from build123d import *

# Parameters (mm, degrees)
F0_W     = 9
F0_H     = 139.6909442604
F0_R     = 1.5
F0_H_2   = 81.4090557396
F1_DEPTH = 10


with BuildPart() as f1:
    # F0 (on Top) → F1 (new body)
    with BuildSketch(Plane.XY):
        with Locations((-251.2277567387, 73.9804314047)):
            Rectangle(F0_W, F0_H)
        with Locations((-251.2277567387, 18.8259035349)):
            Circle(F0_R, mode=Mode.SUBTRACT)
        with Locations((-251.2277567387, 38.8259035349)):
            Circle(F0_R, mode=Mode.SUBTRACT)
        with Locations((-251.2277567387, 58.8259035349)):
            Circle(F0_R, mode=Mode.SUBTRACT)
        with Locations((-251.2277567387, 78.8259035349)):
            Circle(F0_R, mode=Mode.SUBTRACT)
        with Locations((-251.2277567387, 98.8259035349)):
            Circle(F0_R, mode=Mode.SUBTRACT)
        with Locations((-251.2277567387, 118.8259035349)):
            Circle(F0_R, mode=Mode.SUBTRACT)
        with Locations((-251.2277567387, 138.8259035349)):
            Circle(F0_R, mode=Mode.SUBTRACT)
        with BuildLine():
            Line((-246.7277567387, 4.1349592745), (-255.7277567387, 4.1349592745))
            Line((-255.7277567387, 4.1349592745), (-255.7277567387, -3.9008271631))
            ThreePointArc((-255.7277567387, -3.9008271631), (-255.0030118673, -4.4490153217), (-254.7277567387, -5.3150407255))
            ThreePointArc((-254.7277567387, -5.3150407255), (-255.0030118673, -6.1810661293), (-255.7277567387, -6.7292542878))
            Line((-255.7277567387, -6.7292542878), (-255.7277567387, -13.9008271631))
            ThreePointArc((-255.7277567387, -13.9008271631), (-255.0030118673, -14.4490153217), (-254.7277567387, -15.3150407255))
            ThreePointArc((-254.7277567387, -15.3150407255), (-255.0030118673, -16.1810661293), (-255.7277567387, -16.7292542878))
            Line((-255.7277567387, -16.7292542878), (-255.7277567387, -24.7650407255))
            Line((-255.7277567387, -24.7650407255), (-246.7277567387, -24.7650407255))
            Line((-246.7277567387, -24.7650407255), (-246.7277567387, -16.7292542878))
            ThreePointArc((-246.7277567387, -16.7292542878), (-247.7277567387, -15.3150407255), (-246.7277567387, -13.9008271631))
            Line((-246.7277567387, -13.9008271631), (-246.7277567387, -6.7292542878))
            ThreePointArc((-246.7277567387, -6.7292542878), (-247.7277567387, -5.3150407255), (-246.7277567387, -3.9008271631))
            Line((-246.7277567387, -3.9008271631), (-246.7277567387, 4.1349592745))
        make_face()
        with Locations((-251.2277567387, -21.1740964651)):
            Circle(F0_R, mode=Mode.SUBTRACT)
        with Locations((-251.2277567387, -1.1740964651)):
            Circle(F0_R, mode=Mode.SUBTRACT)
        with BuildLine():
            Line((-255.7277567387, -3.9008271631), (-255.7277567387, 4.1349592745))
            Line((-255.7277567387, 4.1349592745), (-261.2277567387, 4.1349592745))
            Line((-261.2277567387, 4.1349592745), (-261.2277567387, -24.7650407255))
            Line((-261.2277567387, -24.7650407255), (-255.7277567387, -24.7650407255))
            Line((-255.7277567387, -24.7650407255), (-255.7277567387, -16.7292542878))
            ThreePointArc((-255.7277567387, -16.7292542878), (-257.7277567387, -15.3150407255), (-255.7277567387, -13.9008271631))
            Line((-255.7277567387, -13.9008271631), (-255.7277567387, -6.7292542878))
            ThreePointArc((-255.7277567387, -6.7292542878), (-257.7277567387, -5.3150407255), (-255.7277567387, -3.9008271631))
        make_face()
        with BuildLine():
            Line((-241.2277567387, 4.1349592745), (-246.7277567387, 4.1349592745))
            Line((-246.7277567387, 4.1349592745), (-246.7277567387, -3.9008271631))
            ThreePointArc((-246.7277567387, -3.9008271631), (-245.3617313349, -4.0902958541), (-244.7277567387, -5.3150407255))
            ThreePointArc((-244.7277567387, -5.3150407255), (-245.3617313349, -6.5397855969), (-246.7277567387, -6.7292542878))
            Line((-246.7277567387, -6.7292542878), (-246.7277567387, -13.9008271631))
            ThreePointArc((-246.7277567387, -13.9008271631), (-245.3617313349, -14.0902958541), (-244.7277567387, -15.3150407255))
            ThreePointArc((-244.7277567387, -15.3150407255), (-245.3617313349, -16.5397855969), (-246.7277567387, -16.7292542878))
            Line((-246.7277567387, -16.7292542878), (-246.7277567387, -24.7650407255))
            Line((-246.7277567387, -24.7650407255), (-241.2277567387, -24.7650407255))
            Line((-241.2277567387, -24.7650407255), (-241.2277567387, 4.1349592745))
        make_face()
        with Locations((-251.2277567387, -65.4695685953)):
            Rectangle(F0_W, F0_H_2)
        with Locations((-251.3328434825, -101.1740964651)):
            Circle(F0_R, mode=Mode.SUBTRACT)
        with Locations((-251.2277567387, -81.1740964651)):
            Circle(F0_R, mode=Mode.SUBTRACT)
        with Locations((-251.2277567387, -61.1740964651)):
            Circle(F0_R, mode=Mode.SUBTRACT)
        with Locations((-251.2277567387, -41.1740964651)):
            Circle(F0_R, mode=Mode.SUBTRACT)
    extrude(amount=F1_DEPTH)


solid = f1.part
Verification items for the finished model (mm, model axes). A direction names the side the tool comes from. Give positions to 0.01 mm unless a question says otherwise; leave off trailing zeros. Order: outer loops, then holes, each group sorted by start corner. A loop starts at its lowest first (then second) coordinate and runs counter-clockwise, first axis right, second up. Notation, with made-up numbers: M -30,-34.5 L -7,-34.5 A32 cw -7,3.5 Z; hole C 41,-23 d1. An arc over 180 degrees is marked long. Answer as a JSON object with one key per item and string values. Group by question number.
1) Cross-section at B-B (z = 3.25). Give the number of separate pieces and of enclosed holes in the cut face, then the cut area to 3 significant figures.
2) Cross-section at A-A (y = -53). Enter the section's corners in (x, z).
3) Access from +Z, -Z, +X, -X, +Y, -Y to the whole of each face (thin tool, end or side, straight path). Record for faces 1 (the face through (-255.728, -66, 5)), 2 (the face through (-258, 4.135, 5)), 3 (the face through (-244, 4.135, 5)), 4 (the face through (-251, 21, 0)), 5 (the face through (-246.728, -66, 5)).
4) Scan lines: line 1 along X through (y, z) = (79, 3.5); line 2 along Y through (x, z) = (-257, 2.25); line 3 along Y through (x, z) = (-245.25, 9.5). Record each from-to range of solid material in increasing order. Write a range as [from, to].
5) Depth check by flat-ended pin: pin 1 Ø2.5 at (x, y) = (-251.23, 138.83) entering from +Z; pin 2 Ø2 at (y, z) = (94, 7.5) entering from -X; pin 3 Ø1.5 at (x, z) = (-259, 1.5) entering from -Y; pin 4 Ø4 at (y, z) = (-62, 2.5) entering from +X. Enter the tip coordinate at first touch or a pass-through.
Result sheet:
{
 "1": {"separate pieces": "1", "enclosed holes": "17", "area": "2,450 mm2"},
 "2": {"outline": "M -255.73,0 L -246.73,0 L -246.73,10 L -255.73,10 Z"},
 "3": {"face 1": "+Z, -Z, -X, -Y", "face 2": "+Z, -Z, -X, +Y", "face 3": "+Z, -Z, +X, +Y", "face 4": "-Z, +X, -X, +Y, -Y", "face 5": "+Z, -Z, +X, -Y"},
 "4": {"line 1": "x = [-255.73, -252.72], [-249.74, -246.73]", "line 2": "y = [-24.77, -16.6], [-14.03, -6.6], [-4.03, 4.13]", "line 3": "y = [-24.77, -16.45], [-14.18, -6.45], [-4.18, 4.13]"},
 "5": {"pin 1": "passes through", "pin 2": "stops at x = -255.73", "pin 3": "stops at y = -24.77", "pin 4": "stops at x = -246.73"}
}
